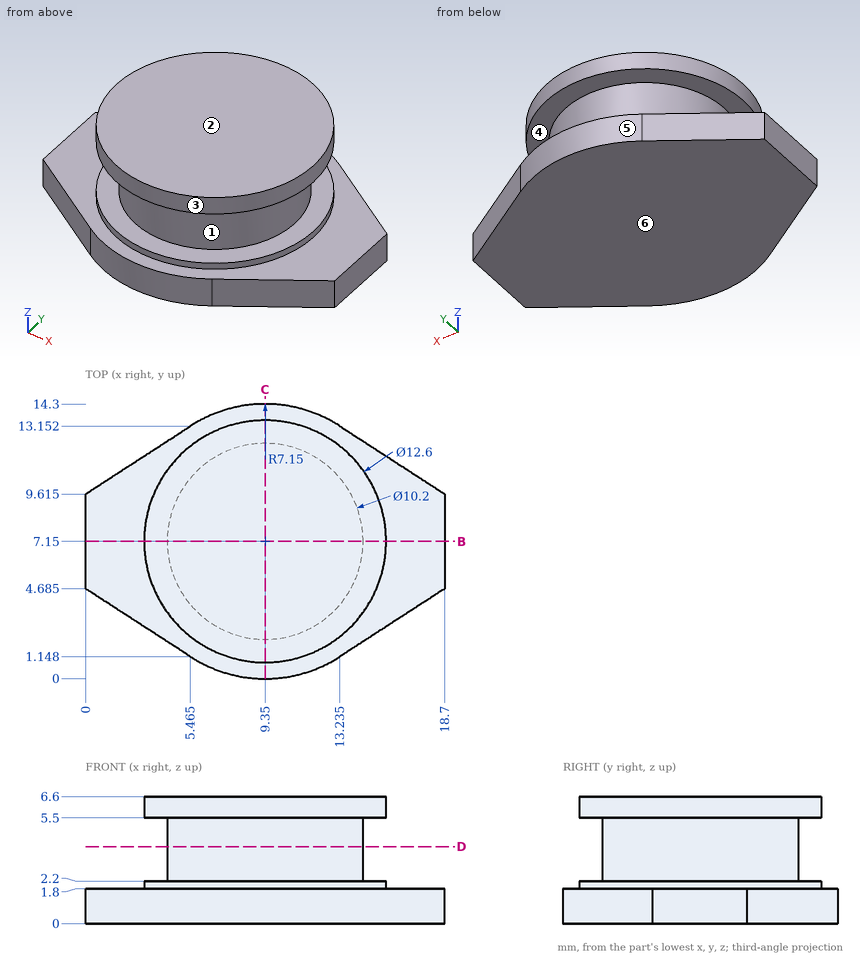
Design review of the part shown in the three views and the two pictorial views. Dimensions are in mm from the part's minimum x, y and z. A direction names the side the tool comes from. Coordinates: 2 decimals unless noted, no trailing zeros. Loops run counter-clockwise (first coordinate to the right, second up) from the corner with the lowest first, then second, coordinate; pieces in that order, holes last.
(1) Consider section D-D, the plane z = 4. Give the boundary of the cut face in (x, y), plus the area to 3 significant figures.
Determined:
outline: circle Ø10.2 at (9.35, 7.15)
area: 81.7 mm2
(2) Insertion check: P1, Ø4, axis at x = 2, y = 2.5, coming from the -Z side; P2, Ø3, axis at x = 7, z = 3.5, coming from the -Y side; P3, Ø1, axis at x = 14, z = 5.5, coming from the -Y side; P4, Ø3, axis at x = 11.5, z = 1.5, coming from the -Y side. Each pin has a flat end and moves straight along its axis. Give the tip position at first contact, or say it passes through.
Determined:
P1: stops at z = 0
P2: stops at y = 1.06
P3: stops at y = 2.41
P4: stops at y = 0.03
(3) Consider section B-B, the plane y = 7.15. Give the boundary of the cut face in (x, z).
Determined:
outline: (0, 0) - (18.7, 0) - (18.7, 1.8) - (15.65, 1.8) - (15.65, 2.2) - (14.45, 2.2) - (14.45, 5.5) - (15.65, 5.5) - (15.65, 6.6) - (3.05, 6.6) - (3.05, 5.5) - (4.25, 5.5) - (4.25, 2.2) - (3.05, 2.2) - (3.05, 1.8) - (0, 1.8) - close
(4) Draft analysis for pull direction Z (two halves, no side actions). For the marked faces 4, 5 and 6, state which applies: +Z half, -Z half, draft (parallel to the pull), parting line (faces both ways), or undercut.
Determined:
face 4: undercut
face 5: draft
face 6: -Z half
(5) Tool access review of the marked faces 1, 2 and 3: name each direction out of +Z, -Z, +X, -X, +Y, -Y from which nothing blocks a thin tool from reaching the whole face with its end or side.
Determined:
face 1: none
face 2: +Z, +X, -X, +Y, -Y
face 3: +Z
(6) Consider section C-C, the plane x = 9.35. Give the boundary of the cut face in (y, z), plus the area to 3 significant figures.
Determined:
outline: (0, 0) - (14.3, 0) - (14.3, 1.8) - (13.45, 1.8) - (13.45, 2.2) - (12.25, 2.2) - (12.25, 5.5) - (13.45, 5.5) - (13.45, 6.6) - (0.85, 6.6) - (0.85, 5.5) - (2.05, 5.5) - (2.05, 2.2) - (0.85, 2.2) - (0.85, 1.8) - (0, 1.8) - close
area: 78.3 mm2
(7) Wall thickness on L1, parallel to Z at x = 4.25, y = 3.75; L2, parallel to Z at x = 17.5, y = 6.25; L3, parallel to Y at x = 13, z = 5.25: over which ranges is each line inside the solid? List them lowest first.
Determined:
L1: z = 0 to 2.2, 5.5 to 6.6
L2: z = 0 to 1.8
L3: y = 3.59 to 10.71
